Check sheet for the modelled part. Datum: model origin and axes. Units: mm. A direction names the side the tool comes from. Round coordinates to 2 decimals unless told otherwise and drop trailing zeros. Loops run counter-clockwise (first coordinate to the right, second up) from the corner with the lowest first, then second, coordinate; pieces in that order, holes last. Notation, with made-up numbers: M 21,-14.75 L 59,-14.75 A28 ccw 59,6.25 Z; hole C 89.25,-38 d1. An arc over 180 degrees is marked long. One line per question, with ' | ' between items. Start each with the question number.
(1) Section check B-B (x = 2.35). Record the boundary of the cut face in (y, z), and give its area (3 significant figures).
(2) Section check A-A (z = 33.5). Record the boundary of the cut face in (x, y).
(3) Go/stop test with flat-tipped pins: P1, Ø1, axis at y = 1.5, z = 28.5, coming from the -X side; P2, Ø3.5, axis at x = 0, y = 0, coming from the +Z side; P3, Ø2.5, axis at x = 0, y = 0, coming from the -Z side. Record where each tip stops, or that it passes through.
(4) Thickness scan on probe 1 along Y at (x, z) = (0, 34.5); probe 2 along X at (y, z) = (0.75, 8.5). Record the ranges inside material, lowest first. Write a range as [from, to].
(5) Tool access check on faces 3 (the face through (-1.29, 0.41, 33.92)), 4 (the face through (1.29, 0.41, 6.08)). Record the directions out of +Z, -Z, +X, -X, +Y, -Y that give a thin tool (end or side, any length) a straight path to the whole face; none if there is none.
(6) Draft check along Y on faces 1 (the face through (-3, 0, 20)), 2 (the face through (-0.224, 0.071, 12.672)). Enter one of: +Y half, -Y half, draft (parallel to the pull), parting line (faces both ways), or undercut.
(7) Section check C-C (x = -2.05). Record the boundary of the cut face in (y, z).
```python
from build123d import *

# Parameters (mm, degrees)
SKETCH1_R                 = 3
BOSS_EXTRUDE1_DEPTH       = 40
F_6_32_TAPPED_HOLE1_D     = 2.7051
F_6_32_TAPPED_HOLE1_DEPTH = 12
F_6_32_TAPPED_HOLE1_TIP   = 0.81269403
F_6_32_TAPPED_HOLE2_D     = 2.7051
F_6_32_TAPPED_HOLE2_DEPTH = 12
F_6_32_TAPPED_HOLE2_TIP   = 0.81269403


with BuildPart() as part:
    # Sketch1 → Boss-Extrude1 (new body)
    with BuildSketch(Plane.XY):
        Circle(SKETCH1_R)
    extrude(amount=BOSS_EXTRUDE1_DEPTH)

    # #6-32 Tapped Hole1
    with Locations(Plane(origin=(0, 0, 0), x_dir=(-1, 0, 0), z_dir=(0, 0, -1))):
        with Locations((0, 0)):
            Hole(F_6_32_TAPPED_HOLE1_D / 2, depth=F_6_32_TAPPED_HOLE1_DEPTH)
            with Locations((0, 0, -(F_6_32_TAPPED_HOLE1_DEPTH + F_6_32_TAPPED_HOLE1_TIP / 2))):  # 118° drill point
                Cone(0, F_6_32_TAPPED_HOLE1_D / 2, F_6_32_TAPPED_HOLE1_TIP, mode=Mode.SUBTRACT)

    # #6-32 Tapped Hole2
    with Locations(Plane.XY.offset(40)):
        with Locations((0, 0)):
            Hole(F_6_32_TAPPED_HOLE2_D / 2, depth=F_6_32_TAPPED_HOLE2_DEPTH)
            with Locations((0, 0, -(F_6_32_TAPPED_HOLE2_DEPTH + F_6_32_TAPPED_HOLE2_TIP / 2))):  # 118° drill point
                Cone(0, F_6_32_TAPPED_HOLE2_D / 2, F_6_32_TAPPED_HOLE2_TIP, mode=Mode.SUBTRACT)


solid = part.part
```
The answers:
1) outline: M -1.86,0 L 1.86,0 L 1.86,40 L -1.86,40 Z | area: 149 mm²
2) outline: C 0,0 d6; hole C 0,0 d2.71
3) P1: x = -2.83 | P2: z = 40 | P3: z = 12.06
4) probe 1: [-3, -1.35], [1.35, 3] | probe 2: [-2.9, -1.13], [1.13, 2.9]
5) face 3: +Z | face 4: -Z
6) face 1: parting line | face 2: undercut
7) outline: M -2.19,0 L 2.19,0 L 2.19,40 L -2.19,40 Z
